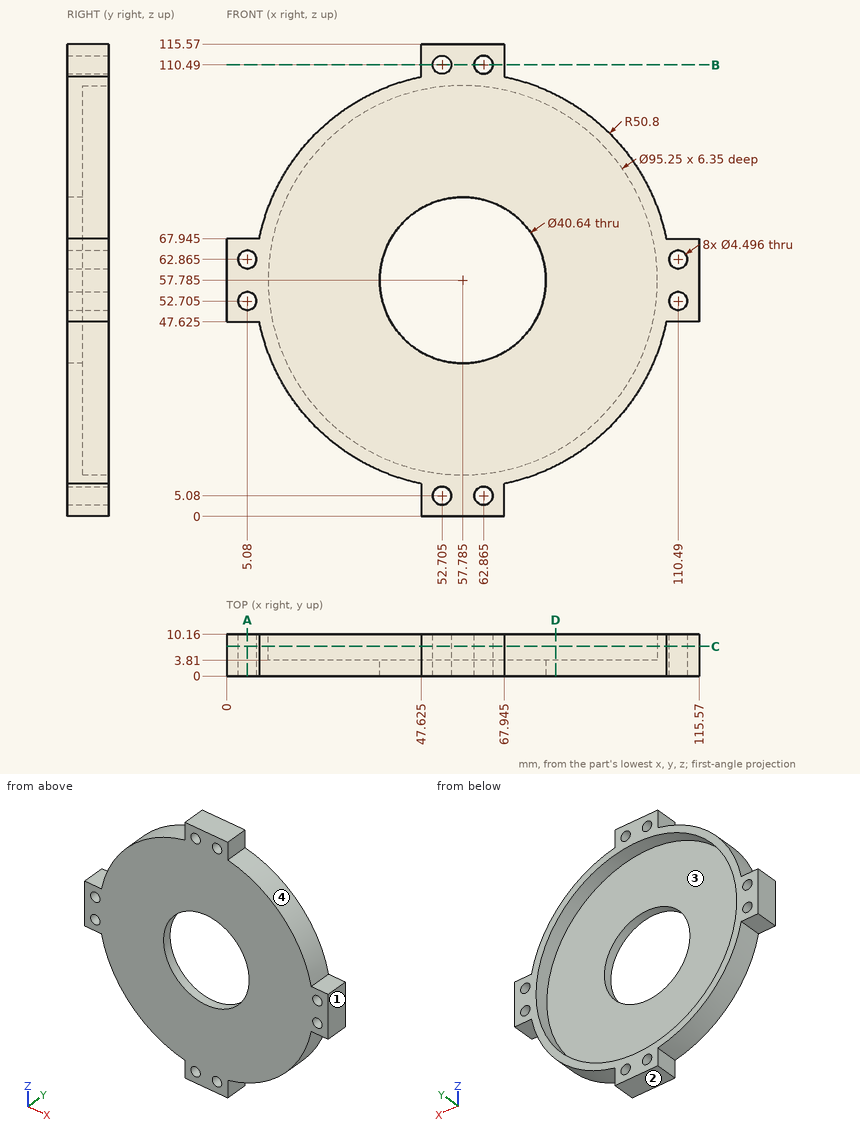
Could you check a few things on this drawing? It's one solid part, dimensions in mm from its lowest x, y, z. Round coordinates to 2 decimals unless told otherwise and drop trailing zeros. Order: outer loops, then holes, each group sorted by start corner. A loop starts at its lowest first (then second) coordinate and runs counter-clockwise, first axis right, second up.
(1) I'm going to push flat-ended pins straight in: pin 1 (10 mm diameter, centred on x = 46, z = 45.5, fed in from -Y); pin 2 (1 mm diameter, centred on x = 24.5, y = 3, fed in from +Z); pin 3 (4 mm diameter, centred on x = 33, z = 20, fed in from +Y); pin 4 (4 mm diameter, centred on y = 4, z = 5, fed in from -X) (3 decimals). Where does each tip first touch, or does it pass through?
Response values:
pin 1: stops at y = 0
pin 2: stops at z = 96.59
pin 3: stops at y = 3.81
pin 4: stops at x = 47.625
(2) Please list where these lines run through material, in increasing order: line 1 along X through (y, z) = (6.5, 5.08) (1 decimal); line 2 along Z through (x, y) = (109.5, 5.5) (1 decimal).
Response values:
line 1: x = 47.6 to 50.5, 55 to 60.6, 65.1 to 67.9
line 2: z = 47.6 to 50.7, 54.7 to 60.8, 64.9 to 67.9
(3) Imagine slicing it at A-A (x = 5.08). Write out the boundary of the cut face in (y, z) (1 decimal), plus the area to 3 significant figures.
Response values:
outline: (0, 47.6) - (10.2, 47.6) - (10.2, 50.5) - (0, 50.5) - close; (0, 55) - (10.2, 55) - (10.2, 60.6) - (0, 60.6) - close; (0, 65.1) - (10.2, 65.1) - (10.2, 67.9) - (0, 67.9) - close
area: 115 mm2
(4) If we mould it in two halves opening along Z, with no side actions, what happens to the marked faces 1, 2, 3 and 4? For each: released by +Z, released by -Z, zero draft, split by the parting line, or undercut.
Response values:
face 1: zero draft
face 2: released by -Z
face 3: undercut
face 4: released by +Z
(5) Imagine slicing it at D-D (x = 80.5). Write out the boundary of the cut face in (y, z).
Response values:
outline: (0, 12.35) - (10.16, 12.35) - (10.16, 15.93) - (3.81, 15.93) - (3.81, 99.64) - (10.16, 99.64) - (10.16, 103.22) - (0, 103.22) - close
(6) Imagine slicing it at C-C (y = 7.25). Count the separate pieces of the cut face and the enclosed holes in it, plus the area to 3 significant figures.
Response values:
separate pieces: 1
enclosed holes: 9
area: 1,450 mm2
(7) Imagine slicing it at B-B (z = 110.49). Write out the boundary of the cut face in (x, y) (1 decimal), plus the area to 3 significant figures.
Response values:
outline: (47.6, 0) - (50.5, 0) - (50.5, 10.2) - (47.6, 10.2) - close; (55, 0) - (60.6, 0) - (60.6, 10.2) - (55, 10.2) - close; (65.1, 0) - (67.9, 0) - (67.9, 10.2) - (65.1, 10.2) - close
area: 115 mm2
